```python
from build123d import *

# Parameters (mm, degrees)
SKETCH1_W           = 76.2
SKETCH1_H           = 25.4
BOSS_EXTRUDE1_DEPTH = 19.05
SKETCH1_7_W         = 25.4
SKETCH1_7_H         = 25.4
BOSS_EXTRUDE3_DEPTH = 31.75
CUT_EXTRUDE4_DEPTH  = 84.521209881
FILLET1_R           = 12.7
SKETCH3_R           = 3.3782
CUT_EXTRUDE5_DEPTH  = 65.757547823
CUT_EXTRUDE6_DEPTH  = 4.445


with BuildPart() as part:
    # Sketch1 → Boss-Extrude1 (new body)
    with BuildSketch(Plane(origin=(0, 0, 0), x_dir=(1, 0, 0), z_dir=(0, 1, 0))):
        Rectangle(SKETCH1_W, SKETCH1_H)
    extrude(amount=BOSS_EXTRUDE1_DEPTH)

    # Sketch1<7> → Boss-Extrude3 (add)
    with BuildSketch(Plane(origin=(0, 0, 0), x_dir=(1, 0, 0), z_dir=(0, 1, 0))):
        with Locations((-25.4, 0)):
            Rectangle(SKETCH1_7_W, SKETCH1_7_H)
        with Locations((25.4, 0)):
            Rectangle(SKETCH1_7_W, SKETCH1_7_H)
    extrude(amount=-BOSS_EXTRUDE3_DEPTH)

    # Sketch2 → Cut-Extrude4 (cut, through all)
    with BuildSketch(Plane.ZY.offset(38.1)):
        with BuildLine():
            ThreePointArc((3.3782, -19.05), (2.388748128, -16.661251872), (0, -15.6718))
            Line((0, -15.6718), (0, -22.4282))
            ThreePointArc((0, -22.4282), (2.388748128, -21.438748128), (3.3782, -19.05))
        make_face()
        with BuildLine():
            Line((0, -22.4282), (0, -15.6718))
            ThreePointArc((0, -15.6718), (-3.3782, -19.05), (0, -22.4282))
        make_face()
    extrude(amount=-CUT_EXTRUDE4_DEPTH, mode=Mode.SUBTRACT)

    # Fillet1
    fillet1_edges = [part.edges().sort_by_distance(p)[0] for p in [
        (-25.4, -31.75, 12.7),
        (25.4, -31.75, 12.7),
        (25.4, -31.75, -12.7),
        (-25.4, -31.75, -12.7),
    ]]
    fillet(fillet1_edges, radius=FILLET1_R - 0.0001)  # a hair under: the kernel refuses the full size

    # Sketch3 → Cut-Extrude5 (cut, through all)
    with BuildSketch(Plane(origin=(0, 19.05, 0), x_dir=(1, 0, 0), z_dir=(0, 1, 0))):
        with Locations(Location((0, 0, 0), (0, 0, 270))):
            Circle(SKETCH3_R)
    extrude(amount=-CUT_EXTRUDE5_DEPTH, mode=Mode.SUBTRACT)

    # Sketch4 → Cut-Extrude6 (cut, symmetric)
    with BuildSketch(Plane(origin=(0, 9.525, 0), x_dir=(-1, 0, 0), z_dir=(0, -1, 0))):
        Polygon((6.599113577, 12.7), (-6.599113577, 12.7), (-6.599113577, 0), (-3.299556788, 5.715), (3.299556788, 5.715), (6.599113577, 0), align=None)
        Polygon((-6.599113577, 0), (-3.299556788, -5.715), (3.299556788, -5.715), (6.599113577, 0), (3.299556788, 5.715), (-3.299556788, 5.715), align=None)
    extrude(amount=CUT_EXTRUDE6_DEPTH, both=True, mode=Mode.SUBTRACT)


solid = part.part
```
Geometry check sheet. Reference: the model listing, model coordinates, mm. A direction names the side the tool comes from. Give positions to 0.01 mm unless a question says otherwise; leave off trailing zeros. Write each loop counter-clockwise with the first axis right and the second up, starting at its lowest first coordinate (ties: lowest second). Pieces come first, ordered by that corner, then holes.
1) Section check A-A, the plane y = -11. Record the boundary of the cut face in (x, z), and give its area (3 significant figures).
2) Gauge pin test, flat ends, axial feed: pin 1 (2 mm diameter, centred on x = 28, z = -6.5, fed in from -Y); pin 2 (4 mm diameter, centred on x = -4.5, z = 9, fed in from -Y); pin 3 (12 mm diameter, centred on x = -20.5, z = -3.5, fed in from -Y); pin 4 (2 mm diameter, centred on x = 0.5, y = 9, fed in from -Z) (3 decimals). Record the tip position at first contact, or that the pin passes through.
3) Release check for a two-part mould opening along Y. For faces 1 (the flat face through (-4.926, 9.463, 2.898)), 2 (the flat face through (38.1, -7, 0)), 3 (the cylindrical face through (25.58, -27.93, 9.08)), 4 (the flat face through (6.599, 9, -6)) record: pulls with the +Y half, pulls with the -Y half, needs draft (parallel to the pull), parting line crosses it, or undercut.
4) Section check C-C, the plane x = 0. Record the boundary of the cut face in (y, z) (3 decimals).
5) Material ranges on L1, parallel to X at y = 16.95, z = 0; L2, parallel to X at y = -14, z = -10.5; L3, parallel to Z at x = -24, y = -20, recorded low to high.
6) Section check D-D, the plane z = -5.25. Record the boundary of the cut face in (x, y).
7) Access from +Z, -Z, +X, -X, +Y, -Y to the whole of each face (thin tool, end or side, straight path). Record for faces 5 (the flat face through (-38.1, -6, 0)), 6 (the flat face through (-12.7, -12, 0)), 7 (the flat face through (-6.599, 9, -6)).
Computed:
1. outline: (-38.1, -12.7) - (-12.7, -12.7) - (-12.7, 12.7) - (-38.1, 12.7) - close; (12.7, -12.7) - (38.1, -12.7) - (38.1, 12.7) - (12.7, 12.7) - close
1. area: 1,290 mm2
2. pin 1: stops at y = -30.5
2. pin 2: stops at y = 0
2. pin 3: stops at y = -31.75
2. pin 4: stops at z = 5.715
3. face 1: undercut
3. face 2: needs draft
3. face 3: pulls with the -Y half
3. face 4: undercut
4. outline: (0, -12.7) - (5.08, -12.7) - (5.08, -3.378) - (0, -3.378) - close; (0, 3.378) - (5.08, 3.378) - (5.08, 5.715) - (13.97, 5.715) - (13.97, 3.378) - (19.05, 3.378) - (19.05, 12.7) - (0, 12.7) - close; (13.97, -12.7) - (19.05, -12.7) - (19.05, -3.378) - (13.97, -3.378) - close
5. L1: x = -38.1 to -3.38, 3.38 to 38.1
5. L2: x = -38.1 to -12.7, 12.7 to 38.1
5. L3: z = -12.66 to -3.24, 3.24 to 12.66
6. outline: (-38.1, -30.61) - (-12.7, -30.61) - (-12.7, 0) - (12.7, 0) - (12.7, -30.61) - (38.1, -30.61) - (38.1, 19.05) - (-38.1, 19.05) - close; hole (-6.6, 5.08) - (6.6, 5.08) - (6.6, 13.97) - (-6.6, 13.97) - close
7. face 5: +Z, -Z, -X, +Y, -Y
7. face 6: +Z, -Z, -Y
7. face 7: -Z
